```python
from build123d import *

# Parameters (mm, degrees)
F0_R     = 4.3303007039
F1_DEPTH = 101.6
F2_W     = 14.3698975444
F2_H     = 23.7585008144


with BuildPart() as f1:
    # F0 (on Right) → F1 (new body, symmetric)
    with BuildSketch(Plane.YZ):
        Circle(F0_R)
    extrude(amount=F1_DEPTH, both=True)

    # F2 (on Front) → F3 (revolve)
    with BuildSketch(Plane.XZ):
        Polygon((-92.3030078411, 50.7372282445), (-92.3030078411, 0), (0, 0), (0, 40.031991899), (0, 50.7372282445), align=None)
        Polygon((0, 40.031991899), (0, 0), (19.8729075491, 0), (19.8729075491, 28.4771621227), (19.8729075491, 40.031991899), align=None)
        Polygon((19.8729075491, 28.4771621227), (19.8729075491, 0), (37.7754718065, 0), (37.7754718065, 23.7585008144), (37.7754718065, 28.4771621227), align=None)
        with Locations((44.9604205787, 11.8792504072)):
            Rectangle(F2_W, F2_H)
    revolve(axis=Axis((0, 0, 0), (1, 0, 0)))


solid = f1.part
```
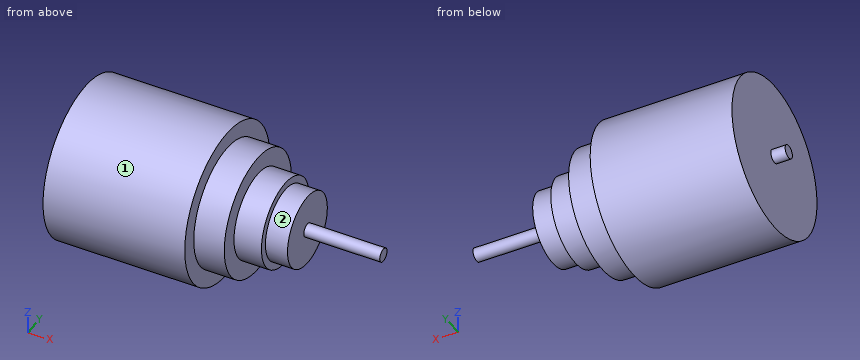
Here's how the part is built. I have some questions about the finished solid (model axes, mm). Face numbers are marked on the shaded views. A direction names the side the tool comes from. Round coordinates to 2 decimals unless told otherwise and drop trailing zeros. Order: outer loops, then holes, each group sorted by start corner. A loop starts at its lowest first (then second) coordinate and runs counter-clockwise, first axis right, second up. Notation, with made-up numbers: M 42,-15 L 81,-15 A31 cw 81,18 Z; hole C 53,26.5 d10. An arc over 180 degrees is marked long. One line per question, with ' | ' between items.
1) I want a section at D-D, the plane z = 31.5. Write out the boundary of the cut face in (x, y), then the cut area to 3 significant figures.
Working result:
outline: M -92.3,-39.77 L 0,-39.77 L 0,-24.7 L 19.87,-24.7 L 19.87,24.7 L 0,24.7 L 0,39.77 L -92.3,39.77 Z | area: 8,320 mm²
2) I want a section at A-A, the plane y = 0. Write out the boundary of the cut face in (x, z), then the cut area to 3 significant figures.
Working result:
outline: M -101.6,-4.33 L -92.3,-4.33 L -92.3,-50.74 L 0,-50.74 L 0,-40.03 L 19.87,-40.03 L 19.87,-28.48 L 37.78,-28.48 L 37.78,-23.76 L 52.15,-23.76 L 52.15,-4.33 L 101.6,-4.33 L 101.6,4.33 L 52.15,4.33 L 52.15,23.76 L 37.78,23.76 L 37.78,28.48 L 19.87,28.48 L 19.87,40.03 L 0,40.03 L 0,50.74 L -92.3,50.74 L -92.3,4.33 L -101.6,4.33 Z | area: 13,200 mm²
3) I need wall thicknesses on line 1 along X through (y, z) = (30, 38); line 2 along X through (y, z) = (-12, 31.5); line 3 along Y through (x, z) = (-35, 0). Which ranges of each line are inside material? Lowest first, please.
Working result:
line 1: -92.3 to 0 | line 2: -92.3 to 19.87 | line 3: -50.74 to 50.74
4) I want a section at C-C, the plane x = -6. Write out the boundary of the cut face in (y, z), then the cut area to 3 significant figures.
Working result:
outline: C 0,0 d101.47 | area: 8,090 mm²
5) For the marked faces 1 and 2, which set-ups out of +Z, -Z, +X, -X, +Y, -Y let a thin tool reach every point of the face, with its end or its side?
Working result:
face 1: +X, -X | face 2: +X
6) I want a section at B-B, the plane z = 8. Write out the boundary of the cut face in (x, y), then the cut area to 3 significant figures.
Working result:
outline: M -92.3,-50.1 L 0,-50.1 L 0,-39.22 L 19.87,-39.22 L 19.87,-27.33 L 37.78,-27.33 L 37.78,-22.37 L 52.15,-22.37 L 52.15,22.37 L 37.78,22.37 L 37.78,27.33 L 19.87,27.33 L 19.87,39.22 L 0,39.22 L 0,50.1 L -92.3,50.1 Z | area: 12,400 mm²
7) For pin 1 Ø12 at (x, y) = (-71, 6) entering from +Z; pin 2 Ø5 at (y, z) = (7.5, 21) entering from +X; pin 3 Ø1 at (y, z) = (5, -38.5) entering from +X; pin 4 Ø10 at (y, z) = (-10.5, -15.5) entering from -X, each with a flat end and sliding along its axis, tell me the tip position at first contact or that it passes through.
Working result:
pin 1: z = 50.74 | pin 2: x = 52.15 | pin 3: x = 19.87 | pin 4: x = -92.3
